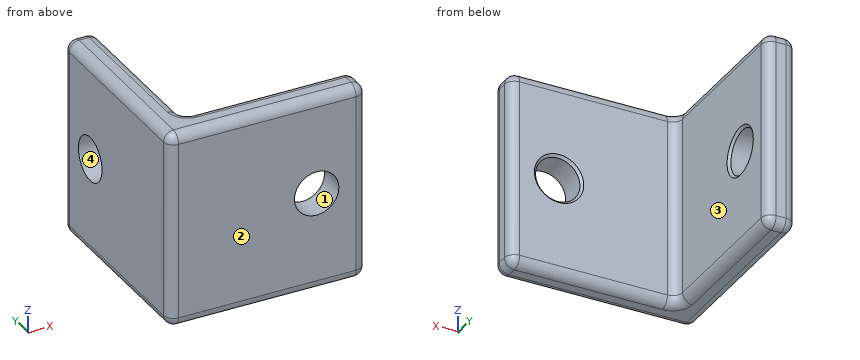
Autodesk Inventor part; units mm, degrees
ref_plane "YZ Plane" through (0, 0, 0) normal (1, 0, 0) x (0, 1, 0)
ref_plane "XZ Plane" through (0, 0, 0) normal (0, 1, 0) x (-1, 0, 0)
ref_plane "XY Plane" through (0, 0, 0) normal (0, 0, 1) x (1, 0, 0)
sketch "Esquisse1" plane through (0, 0, 0) normal (0, 1, 0) x (-1, 0, 0)
  line L0 (-10, 10) -> (10, 10)
  line L1 (10, 10) -> (10, -10)
  line L2 (10, -10) -> (-10, -10)
  line L3 (-10, -10) -> (-10, 10)
  line L4 (-10, 10) -> (10, -10) construction
  line L5 (10, 10) -> (-10, -10) construction
  point P0 (0, 0)
  dimension "d0" = 20
  dimension "d1" = 20
extrude "Extrusion1" add sketch "Esquisse1" along normal blind 3
sketch "Esquisse2" plane through (-10, 0, -10) normal (-1, 0, 0) x (0, 0, 1)
  line L0 (0, 20) -> (20, 20)
  line L1 (20, 20) -> (20, 3)
  line L2 (20, 3) -> (0, 3)
  line L3 (0, 3) -> (0, 20)
  line L4 (0, 20) -> (20, 3) construction
  line L5 (20, 20) -> (0, 3) construction
  line L6 (0, 0) -> (20, 0)
  point P0 (10, 0)
  point P1 (10, 11.5)
  dimension "d4" = 20
  dimension "d5" = 17
  dimension "d6" = 3
extrude "Extrusion2" add sketch "Esquisse2" against normal blind 3
fillet "Congé1" radius 1 18 edges at (10, 3, 0) (1.5, 3, 10) (10, 1.5, 10) (-7, 11.5, 10) (0, 0, 10) (-10, 10, 10) (-10, 0, 0) (-10, 10, -10) (0, 0, -10) (1.5, 3, -10) (-7, 11.5, -10) (10, 1.5, -10) (10, 0, 0) (-7, 3, 0) (-7, 20, 0) (-10, 20, 0) (-8.5, 20, 10) (-8.5, 20, -10)
sketch "Esquisse3" plane through (0, 3, 0) normal (0, 1, 0) x (1, 0, 0)
  line L0 (10, -9) -> (10, 9)
  point P0 (0, 0)
  point P1 (5, -0.0654)
  dimension "d24" = 5
hole "Perçage1" at (5, 3, 0.0654) direction (0, -1, 0) diameter 4.5 depth 16.2 tip angle 118 countersink diameter 5 countersink angle 90
sketch "Esquisse4" plane through (-7, 0, -10) normal (1, 0, 0) x (0, 0, -1)
  line L0 (-1, 20) -> (-19, 20)
  line L1 (-20, 19) -> (-20, 4)
  point P0 (-10, 0)
  point P1 (-10, 15)
  dimension "d25" = 5
  dimension "d26" = 10
hole "Perçage2" at (-7, 15, 0) direction (-1, 0, 0) diameter 4.5 depth 16.2 tip angle 118 countersink diameter 5 countersink angle 90
properties part number "Aquerre"
Source: CAD feature listing. Evaluate the final solid. Frame: model axes, mm. Face numbers are marked on the shaded views. A direction names the side the tool comes from. Round coordinates to 2 decimals unless told otherwise and drop trailing zeros. Write each loop counter-clockwise with the first axis right and the second up, starting at its lowest first coordinate (ties: lowest second). Pieces come first, ordered by that corner, then holes. Notation, with made-up numbers: (54.5, -5.75) - (103.5, -5.75) arc R22 ccw to (103.5, 6.25) - close; hole circle Ø11 at (83.25, 44.5). An arc over 180 degrees is marked (long way). Use CSV: the item, a comma, the result in double quotes. Start each with the question number.
(1) Mould query, pull axis Z, two halves, no side actions, for the marked faces 1 and 2. Classes: pulls with the +Z half, pulls with the -Z half, needs draft (parallel to the pull), parting line crosses it, or undercut.
(2) Cut plane C-C, the plane z = -7. Return loops of the section in (x, y).
(3) Cut plane B-B, the plane y = 15. Return loops of the section in (x, z).
(4) First-contact query: pin 1 Ø2 at (x, z) = (-2.5, -2.5) entering from +Y; pin 2 Ø3.5 at (x, z) = (5, 0.07) entering from +Y; pin 3 Ø8 at (x, y) = (5, 6.5) entering from -Z; pin 4 Ø4.5 at (y, z) = (14.5, 2.5) entering from +X. Flat tips, straight axial feed; report the tip coordinate or a pass-through.
(5) Material intervals for probe 1 along Y at (x, z) = (-7.95, 0); probe 2 along Z at (x, y) = (-9.05, 15); probe 3 along Z at (x, y) = (5, 1.9), sorted ascending. Write a range as [from, to].
(6) Cut plane A-A, the plane x = 5. Return loops of the section in (y, z), and give its area (3 significant figures).
(7) Cut plane D-D, the plane x = -4.25. Return loops of the section in (y, z).
(8) Set-up query: the marked faces 3 and 4. Return all of +Z, -Z, +X, -X, +Y, -Y with unobstructed straight access to the full face (end or side cutting, diameter ignored); none if empty.
Geometry says:
1,face 1,"undercut"
1,face 2,"needs draft"
2,outline,"(-10, 1) arc R1 ccw to (-9, 0) - (9, 0) arc R1 ccw to (10, 1) - (10, 2) arc R1 ccw to (9, 3) - (-6, 3) arc R1 cw to (-7, 4) - (-7, 19) arc R1 ccw to (-8, 20) - (-9, 20) arc R1 ccw to (-10, 19) - close"
3,outline,"(-10, -9) arc R1 ccw to (-9, -10) - (-8, -10) arc R1 ccw to (-7, -9) - (-7, -2.5) - (-7.25, -2.25) - (-10, -2.25) - close; (-10, 2.25) - (-7.25, 2.25) - (-7, 2.5) - (-7, 9) arc R1 ccw to (-8, 10) - (-9, 10) arc R1 ccw to (-10, 9) - close"
4,pin 1,"y = 3"
4,pin 2,"through"
4,pin 3,"z = -9.87"
4,pin 4,"x = -7"
5,probe 1,"[0, 12.75], [17.25, 20]"
5,probe 2,"[-10, -2.25], [2.25, 10]"
5,probe 3,"[-10, -2.18], [2.32, 10]"
6,outline,"(0, -9) arc R1 ccw to (1, -10) - (2, -10) arc R1 ccw to (3, -9) - (3, -2.43) - (2.75, -2.18) - (0, -2.18) - close; (0, 2.32) - (2.75, 2.32) - (3, 2.57) - (3, 9) arc R1 ccw to (2, 10) - (1, 10) arc R1 ccw to (0, 9) - close"
6,area,"45.6 mm²"
7,outline,"(0, -9) arc R1 ccw to (1, -10) - (2, -10) arc R1 ccw to (3, -9) - (3, 9) arc R1 ccw to (2, 10) - (1, 10) arc R1 ccw to (0, 9) - close"
8,face 3,"+Z, -Z, +X, +Y"
8,face 4,"+X, -X"
